Read the model definition and answer for the solid it produces. Units are mm, in the model's axes. A direction names the side the tool comes from. Coordinates: 2 decimals unless noted, no trailing zeros. Write each loop counter-clockwise with the first axis right and the second up, starting at its lowest first coordinate (ties: lowest second). Pieces come first, ordered by that corner, then holes.
1) Each of these flat-tipped pins is pushed along its axis until it touches: pin 1 Ø6.5 at (x, z) = (10, -81.5) entering from +Y; pin 2 Ø2 at (x, y) = (77.5, 1.5) entering from +Z; pin 3 Ø1.5 at (x, y) = (38, 8.5) entering from -Z. Where does it stop, or does it pass through?
2) The part is cut by section D-D (x = 55.1). Determine the outline of the cut face in (y, z), then the cut area to 3 significant figures.
3) The part is cut by section C-C (x = 11). Determine the outline of the cut face in (y, z), then the cut area to 3 significant figures.
4) Which of the six approach directions +Z, -Z, +X, -X, +Y, -Y give full straight-line access (tool end or side, diameter ignored) to faces 1 (the face through (39.909, 5.472, -46.115)), 2 (the face through (0, 4, -25)), 3 (the face through (21.734, 6.121, -47.974))?
5) The part is cut by section B-B (z = -7). Determine the outline of the cut face in (x, y) (3 decimals), then the cut area to 3 significant figures.
6) Determine the mould class of faces 4 (the face through (53.79, 3.75, -86.5)), 5 (the face through (67, 4, -51)), 6 (the face through (4, 11.1, -53)) for opening direction Z: +Z half, -Z half, draft (parallel to the pull), parting line (faces both ways), or undercut.
7) Find the intervals of material crossed by line 1 (X direction, y = 0.9, z = -82); line 2 (X direction, y = 6.6, z = -82); line 3 (Z direction, x = 66, y = 5.25), in increasing order.
8) The part is cut by section A-A (y = 9.5). Give the number of separate pieces and of enclosed holes in the cut face, then the cut area to 3 significant figures.
from build123d import *

# Parameters (mm, degrees)
SKETCH1_W           = 11
SKETCH1_H           = 1
SKETCH1_W_2         = 101.6
SKETCH1_W_3         = 46.35
SKETCH1_R           = 1.65
BOSS_EXTRUDE1_DEPTH = 7.6
SKETCH2_R           = 3
CUT_EXTRUDE1_DEPTH  = 3
SKETCH3_R           = 3
SKETCH3_R_2         = 1.65
BOSS_EXTRUDE3_DEPTH = 3.5


with BuildPart() as part:
    # Sketch1 → Boss-Extrude1 (new body)
    with BuildSketch(Plane(origin=(0, 0, 0), x_dir=(1, 0, 0), z_dir=(0, 1, 0))):
        with Locations((-5.5, 51.5)):
            Rectangle(SKETCH1_W, SKETCH1_H)
        with Locations((39.8, 105.8)):
            Rectangle(SKETCH1_W_2, SKETCH1_H)
        with Locations((67.425, 51.5)):
            Rectangle(SKETCH1_W_3, SKETCH1_H)
        Polygon((-11, 52), (-11, 105.3), (90.6, 105.3), (90.6, 52), (44.25, 52), (44.25, 0), (0, 0), (0, 52), align=None)
        with Locations((22.125, 7)):
            Circle(SKETCH1_R, mode=Mode.SUBTRACT)
        with Locations((22.125, 45)):
            Circle(SKETCH1_R, mode=Mode.SUBTRACT)
        with Locations((66, 82)):
            Circle(SKETCH1_R, mode=Mode.SUBTRACT)
        with Locations((11, 82)):
            Circle(SKETCH1_R, mode=Mode.SUBTRACT)
        with Locations((41.125, 7)):
            Circle(SKETCH1_R, mode=Mode.SUBTRACT)
        with Locations((3.125, 7)):
            Circle(SKETCH1_R, mode=Mode.SUBTRACT)
        with Locations((41.125, 45)):
            Circle(SKETCH1_R, mode=Mode.SUBTRACT)
        with Locations((3.125, 45)):
            Circle(SKETCH1_R, mode=Mode.SUBTRACT)
        with Locations((85.55, 54.5)):
            Circle(SKETCH1_R, mode=Mode.SUBTRACT)
        with Locations((55.1, 59.6)):
            Circle(SKETCH1_R, mode=Mode.SUBTRACT)
        with Locations((55.1, 87.5)):
            Circle(SKETCH1_R, mode=Mode.SUBTRACT)
        with Locations((3, 54.5)):
            Circle(SKETCH1_R, mode=Mode.SUBTRACT)
        with Locations((79.2, 102.7)):
            Circle(SKETCH1_R, mode=Mode.SUBTRACT)
        with Locations((4.3, 102.7)):
            Circle(SKETCH1_R, mode=Mode.SUBTRACT)
    extrude(amount=BOSS_EXTRUDE1_DEPTH)

    # Sketch2 → Cut-Extrude1 (cut)
    with BuildSketch(Plane(origin=(0, 7.6, 0), x_dir=(1, 0, 0), z_dir=(0, 1, 0))):
        with Locations((11, 82)):
            Circle(SKETCH2_R)
        with Locations((66, 82)):
            Circle(SKETCH2_R)
        with Locations((22.125, 45)):
            Circle(SKETCH2_R)
        with Locations((22.125, 7)):
            Circle(SKETCH2_R)
    extrude(amount=-CUT_EXTRUDE1_DEPTH, mode=Mode.SUBTRACT)

    # Sketch3 → Boss-Extrude3 (add)
    with BuildSketch(Plane(origin=(0, 7.6, 0), x_dir=(1, 0, 0), z_dir=(0, 1, 0))):
        with Locations((3.125, 7)):
            Circle(SKETCH3_R)
        with Locations((3.125, 7)):
            Circle(SKETCH3_R_2, mode=Mode.SUBTRACT)
        with Locations((41.125, 7)):
            Circle(SKETCH3_R)
        with Locations((41.125, 7)):
            Circle(SKETCH3_R_2, mode=Mode.SUBTRACT)
        with Locations((3.125, 45)):
            Circle(SKETCH3_R)
        with Locations((3.125, 45)):
            Circle(SKETCH3_R_2, mode=Mode.SUBTRACT)
        with Locations((41.125, 45)):
            Circle(SKETCH3_R)
        with Locations((41.125, 45)):
            Circle(SKETCH3_R_2, mode=Mode.SUBTRACT)
        with Locations((3, 54.5)):
            Circle(SKETCH3_R)
        with Locations((3, 54.5)):
            Circle(SKETCH3_R_2, mode=Mode.SUBTRACT)
        with Locations((55.1, 59.6)):
            Circle(SKETCH3_R)
        with Locations((55.1, 59.6)):
            Circle(SKETCH3_R_2, mode=Mode.SUBTRACT)
        with Locations((85.55, 54.5)):
            Circle(SKETCH3_R)
        with Locations((85.55, 54.5)):
            Circle(SKETCH3_R_2, mode=Mode.SUBTRACT)
        with Locations((79.2, 102.7)):
            Circle(SKETCH3_R)
        with Locations((79.2, 102.7)):
            Circle(SKETCH3_R_2, mode=Mode.SUBTRACT)
        with Locations((4.3, 102.7)):
            Circle(SKETCH3_R)
        with Locations((4.3, 102.7)):
            Circle(SKETCH3_R_2, mode=Mode.SUBTRACT)
    extrude(amount=BOSS_EXTRUDE3_DEPTH)


solid = part.part
Reported:
1. pin 1: stops at y = 7.6
1. pin 2: stops at z = -51
1. pin 3: stops at z = -46.83
2. outline: (0, -106.3) - (7.6, -106.3) - (7.6, -89.15) - (0, -89.15) - close; (0, -85.85) - (7.6, -85.85) - (7.6, -62.6) - (11.1, -62.6) - (11.1, -61.25) - (0, -61.25) - close; (0, -57.95) - (11.1, -57.95) - (11.1, -56.6) - (7.6, -56.6) - (7.6, -51) - (0, -51) - close
2. area: 380 mm2
3. outline: (0, -106.3) - (7.6, -106.3) - (7.6, -85) - (4.6, -85) - (4.6, -83.65) - (0, -83.65) - close; (0, -80.35) - (4.6, -80.35) - (4.6, -79) - (7.6, -79) - (7.6, 0) - (0, 0) - close
3. area: 775 mm2
4. face 1: +Y, -Y
4. face 2: +Z, -X, +Y, -Y
4. face 3: +Y
5. outline: (0, 0) - (1.475, 0) - (1.475, 11.1) - (0.125, 11.1) - (0.125, 7.6) - (0, 7.6) - close; (4.775, 0) - (20.475, 0) - (20.475, 4.6) - (19.125, 4.6) - (19.125, 7.6) - (6.125, 7.6) - (6.125, 11.1) - (4.775, 11.1) - close; (23.775, 0) - (39.475, 0) - (39.475, 11.1) - (38.125, 11.1) - (38.125, 7.6) - (25.125, 7.6) - (25.125, 4.6) - (23.775, 4.6) - close; (42.775, 0) - (44.25, 0) - (44.25, 7.6) - (44.125, 7.6) - (44.125, 11.1) - (42.775, 11.1) - close
5. area: 272 mm2
6. face 4: undercut
6. face 5: +Z half
6. face 6: draft
7. line 1: x = -11 to 9.35, 12.65 to 64.35, 67.65 to 90.6
7. line 2: x = -11 to 8, 14 to 63, 69 to 90.6
7. line 3: z = -106.3 to -85, -79 to -51
8. separate pieces: 9
8. enclosed holes: 9
8. area: 177 mm2
